Design review of the part built by this model. Coordinates are the model's own, in mm. A direction names the side the tool comes from. Coordinates: 2 decimals unless noted, no trailing zeros. Loops run counter-clockwise (first coordinate to the right, second up) from the corner with the lowest first, then second, coordinate; pieces in that order, holes last. Notation, with made-up numbers: (27.5, 77.25) -> (37.5, 77.25) arc R18 cw to (37.5, 94.25) -> close; hole circle Ø4 at (22.25, -8). An arc over 180 degrees is marked (long way). Answer in a Markdown table with one row per item.
Autodesk Inventor part; units mm, degrees
ref_plane "YZ Plane" through (0, 0, 0) normal (1, 0, 0) x (0, 1, 0)
ref_plane "XZ Plane" through (0, 0, 0) normal (0, 1, 0) x (-1, 0, 0)
ref_plane "XY Plane" through (0, 0, 0) normal (0, 0, 1) x (1, 0, 0)
sketch "Sketch1" plane through (0, 0, 0) normal (0, 0, 1) x (1, 0, 0)
  line L0 (0, -22.4) -> (0, 22.4) construction
  line L1 (-22.4, 0) -> (22.4, 0) construction
  line L2 (-16, 16) -> (16, 16)
  line L3 (16, 16) -> (16, -16)
  line L4 (16, -16) -> (-16, -16)
  line L5 (-16, -16) -> (-16, 16)
  line L6 (16, 8) -> (-16, 8)
  line L7 (8, 8) -> (8, -8)
  line L8 (-16, -8) -> (16, -8)
  line L9 (-16, 8) -> (8, 16)
  line L10 (-16, -8) -> (8, -16)
  line L11 (8, -8) -> (16, -16) construction
  line L12 (8, 8) -> (16, 16) construction
  line L13 (-8, 8) -> (-8, -8)
  line L14 (-4, 4) -> (4, 4) construction
  line L15 (4, 4) -> (4, -4) construction
  line L16 (4, -4) -> (-4, -4) construction
  line L17 (-4, -4) -> (-4, 4) construction
  circle A0 centre (-4, 4) radius 2.5
  circle A1 centre (4, 4) radius 2.5
  circle A2 centre (4, -4) radius 2.5
  circle A3 centre (-4, -4) radius 2.5
  circle A4 centre (12, 12) radius 2.5
  circle A5 centre (12, -12) radius 2.5
  line L18 (9.5, -14.5) -> (14.5, -14.5)
  line L19 (14.5, -14.5) -> (14.5, -9.5)
  line L20 (14.5, -9.5) -> (9.5, -9.5)
  line L21 (9.5, -9.5) -> (9.5, -14.5)
  line L22 (9.5, 9.5) -> (14.5, 9.5)
  line L23 (14.5, 9.5) -> (14.5, 14.5)
  line L24 (14.5, 14.5) -> (9.5, 14.5)
  line L25 (9.5, 14.5) -> (9.5, 9.5)
  point P0 (-16, 0)
  point P1 (0, 16)
  point P2 (8, 0)
  point P3 (0, 4)
  point P4 (4, 0)
  dimension "d0" = 32
  dimension "d1" = 32
  dimension "d2" = 8
  dimension "d3" = 16
  dimension "d4" = 16
  dimension "d5" = 8
  dimension "d6" = 5
extrude "Extrusion1" add sketch "Sketch1" along normal blind 9.6 contours L2 L3 L6 L9 | L8 L3 L4 L10 | A4 | L23 L22 A4 | A4 L24 L23 | A4 L25 L24 | L22 L25 A4 | A5 | L19 L18 A5 | A5 L20 L19 | A5 L21 L20 | L18 L21 A5
extrude "Extrusion5" add sketch "Sketch1" along normal blind 6.4 contours L6 L7 L8 L13 | A0 | A1 | A2 | A3
extrude "Extrusion6" add sketch "Sketch1" along normal blind 8 contours A0 | A1 | A2 | A3
extrude "Extrusion7" add sketch "Sketch1" along normal blind 11.2 contours A4 | A5
extrude "Extrusion8" cut sketch "Sketch1" along normal blind 1.6 contours A4 | L23 L22 A4 | A4 L24 L23 | A4 L25 L24 | L22 L25 A4 | A5 | L19 L18 A5 | A5 L20 L19 | A5 L21 L20 | L18 L21 A5
properties part number "LEGO Brick 2399" material "Steel"
(1) Take a section at C-C on x = -4. Give the boundary of the cut face in (y, z), and give its area (3 significant figures).
Evaluation:
| item | result |
|---|---|
| outline | (-12, 0) -> (12, 0) -> (12, 9.6) -> (8, 9.6) -> (8, 6.4) -> (6.5, 6.4) -> (6.5, 8) -> (1.5, 8) -> (1.5, 6.4) -> (-1.5, 6.4) -> (-1.5, 8) -> (-6.5, 8) -> (-6.5, 6.4) -> (-8, 6.4) -> (-8, 9.6) -> (-12, 9.6) -> close |
| area | 195 mm² |
(2) Tool access review of faces 1 (the flat face through (-8, 0, 3)), 2 (the flat face through (4, -4, 8)), 3 (the flat face through (12, -12, 1.6)), 4 (the cylindrical face through (11.46, -9.56, 10.39)), 5 (the flat face through (8, 0, 3)): name each direction out of +Z, -Z, +X, -X, +Y, -Y from which nothing blocks a thin tool from reaching the whole face with its end or side.
Evaluation:
| item | result |
|---|---|
| face 1 | +Z, -Z, -X |
| face 2 | +Z, +X, -X |
| face 3 | -Z |
| face 4 | +Z |
| face 5 | +Z, -Z, +X |
(3) Take a section at A-A on x = 13.5. Give the boundary of the cut face in (y, z).
Evaluation:
| item | result |
|---|---|
| outline | (-16, 0) -> (-14.5, 0) -> (-14.5, 1.6) -> (-9.5, 1.6) -> (-9.5, 0) -> (-8, 0) -> (-8, 9.6) -> (-10, 9.6) -> (-10, 11.2) -> (-14, 11.2) -> (-14, 9.6) -> (-16, 9.6) -> close; (8, 0) -> (9.5, 0) -> (9.5, 1.6) -> (14.5, 1.6) -> (14.5, 0) -> (16, 0) -> (16, 9.6) -> (14, 9.6) -> (14, 11.2) -> (10, 11.2) -> (10, 9.6) -> (8, 9.6) -> close |
(4) For pin 1 (4 mm diameter, centred on x = 1, y = -10.5, fed in from +Z); pin 2 (5.5 mm diameter, centred on x = -3.5, y = 5, fed in from +Z); pin 3 (3 mm diameter, centred on y = -1.5, z = 2, fed in from -X), all flat-tipped, find the tip position at first contact; note any pin that passes through.
Evaluation:
| item | result |
|---|---|
| pin 1 | stops at z = 9.6 |
| pin 2 | stops at z = 8 |
| pin 3 | stops at x = -8 |
(5) Take a section at B-B on y = -4. Give the boundary of the cut face in (x, z), and give its area (3 significant figures).
Evaluation:
| item | result |
|---|---|
| outline | (-8, 0) -> (8, 0) -> (8, 6.4) -> (6.5, 6.4) -> (6.5, 8) -> (1.5, 8) -> (1.5, 6.4) -> (-1.5, 6.4) -> (-1.5, 8) -> (-6.5, 8) -> (-6.5, 6.4) -> (-8, 6.4) -> close |
| area | 118 mm² |
(6) Draft analysis for pull direction X (two halves, no side actions). For faces 6 (the flat face through (9.5, -12, 1)), 7 (the flat face through (12, -12, 11.2)), 8 (the flat face through (16, -12, 5)), state which applies: pulls with the +X half, pulls with the -X half, needs draft (parallel to the pull), parting line crosses it, or undercut.
Evaluation:
| item | result |
|---|---|
| face 6 | undercut |
| face 7 | needs draft |
| face 8 | pulls with the +X half |
(7) To check wall thickness, follow probe 1 along Y at (x, z) = (9, 5.5); probe 2 along Y at (x, z) = (3.5, 7); probe 3 along Z at (x, y) = (4, 3.5). State the ranges of each line that lie inside material, in increasing order.
Evaluation:
| item | result |
|---|---|
| probe 1 | y = -16 to -8, 8 to 16 |
| probe 2 | y = -14.5 to -8, -6.45 to -1.55, 1.55 to 6.45, 8 to 14.5 |
| probe 3 | z = 0 to 8 |
(8) Take a section at D-D on z = 10.75. Give the boundary of the cut face in (x, y), and give its area (3 significant figures).
Evaluation:
| item | result |
|---|---|
| outline | circle Ø5 at (12, -12); circle Ø5 at (12, 12) |
| area | 39.3 mm² |
